Build history of the part. All positions in model axes, mm. A direction names the side the tool comes from. Give positions to 0.01 mm unless a question says otherwise; leave off trailing zeros. Order: outer loops, then holes, each group sorted by start corner. A loop starts at its lowest first (then second) coordinate and runs counter-clockwise, first axis right, second up. Notation, with made-up numbers: (41.25, 4.25) -> (76.25, 4.25) arc R13 ccw to (76.25, 10.25) -> close; hole circle Ø4 at (65.5, 72.5). An arc over 180 degrees is marked (long way). One line per item, written item: value. Start each with the question number.
(1) Saw through at D-D on x = 4.5. Give the cut face in (y, z), plus the area to 3 significant figures.
(2) Saw through at A-A on x = 0. Give the cut face in (y, z).
(3) Pin check, flat tips, straight feed: pin 1 (0.8 mm diameter, centred on x = -1, y = 1, fed in from +Z); pin 2 (1.8 mm diameter, centred on x = 7, z = -2, fed in from +Y); pin 3 (4 mm diameter, centred on x = 0, z = 0, fed in from +Y). Stop position of each tip, or through.
(4) Probe line 1 (X direction, y = 1.05, z = 2); line 2 (Y direction, x = 0.5, z = 0.5). List the from-to ranges inside material, lowest first.
(5) Which spindle directions (+Z, -Z, +X, -X, +Y, -Y) get a long thin tool onto all of the face, cutting with end or side? Do faces 3 (the flat face through (0, 0, 0)), 4 (the flat face through (7, 0.152, 3)), 5 (the flat face through (-7, 0.152, 0)). Say none if no direction does.
(6) Two-plate mould, pull along X, no slides. Class faces 1 (the flat face through (0, 1.651, 0)), 2 (the flat face through (7, 0.152, -3)): +X half, -X half, draft (parallel to the pull), parting line (faces both ways), or undercut.
```python
from build123d import *

# Parameters (mm, degrees)
SKETCH1_W           = 16.6116
SKETCH1_H           = 9.9568
BOSS_EXTRUDE1_DEPTH = 0.127
SKETCH3_W           = 4.953
SKETCH3_H           = 4.953
BOSS_EXTRUDE3_DEPTH = 1.651
SKETCH4_W           = 2.258810151
SKETCH4_H           = 1.651
BOSS_EXTRUDE4_DEPTH = 0.0254
SKETCH5_R           = 2.348345572
CUT_EXTRUDE1_DEPTH  = 0.127


with BuildPart() as part:
    # Sketch1 → Boss-Extrude1 (new body)
    with BuildSketch(Plane(origin=(0, 0, 0), x_dir=(1, 0, 0), z_dir=(0, 1, 0))):
        Rectangle(SKETCH1_W, SKETCH1_H)
    extrude(amount=BOSS_EXTRUDE1_DEPTH)

    # Sketch3 → Boss-Extrude3 (add)
    with BuildSketch(Plane(origin=(0, 0.127, 0), x_dir=(1, 0, 0), z_dir=(0, 1, 0))):
        Rectangle(SKETCH3_W, SKETCH3_H)
    extrude(amount=BOSS_EXTRUDE3_DEPTH)

    # Sketch4 → Boss-Extrude4 (add)
    with BuildSketch(Plane(origin=(0, 0.127, 0), x_dir=(1, 0, 0), z_dir=(0, 1, 0))):
        with Locations((-7.176394925, 0)):
            Rectangle(SKETCH4_W, SKETCH4_H)
        with Locations((-7.176394925, 2.54)):
            Rectangle(SKETCH4_W, SKETCH4_H)
        with Locations((-7.176394925, -2.54)):
            Rectangle(SKETCH4_W, SKETCH4_H)
        with Locations((7.176394925, -2.54)):
            Rectangle(SKETCH4_W, SKETCH4_H)
        with Locations((7.176394925, 0)):
            Rectangle(SKETCH4_W, SKETCH4_H)
        with Locations((7.176394925, 2.54)):
            Rectangle(SKETCH4_W, SKETCH4_H)
    extrude(amount=BOSS_EXTRUDE4_DEPTH)

    # Sketch5 → Cut-Extrude1 (cut)
    with BuildSketch(Plane(origin=(0, 1.778, 0), x_dir=(1, 0, 0), z_dir=(0, 1, 0))):
        Circle(SKETCH5_R)
    extrude(amount=-CUT_EXTRUDE1_DEPTH, mode=Mode.SUBTRACT)


solid = part.part
```
Results below:
1. outline: (0, -4.98) -> (0.13, -4.98) -> (0.13, 4.98) -> (0, 4.98) -> close
1. area: 1.26 mm²
2. outline: (0, -4.98) -> (0.13, -4.98) -> (0.13, -2.48) -> (1.78, -2.48) -> (1.78, -2.35) -> (1.65, -2.35) -> (1.65, 2.35) -> (1.78, 2.35) -> (1.78, 2.48) -> (0.13, 2.48) -> (0.13, 4.98) -> (0, 4.98) -> close
3. pin 1: stops at z = 2.48
3. pin 2: stops at y = 0.15
3. pin 3: stops at y = 1.65
4. line 1: x = -2.48 to 2.48
4. line 2: y = 0 to 1.65
5. face 3: +Z, -Z, +X, -X, -Y
5. face 4: +Z, -Z, +X, +Y
5. face 5: +Z, -Z, -X, +Y
6. face 1: undercut
6. face 2: draft
